Build history of the part. All positions in model axes, mm. A direction names the side the tool comes from. Give positions to 0.01 mm unless a question says otherwise; leave off trailing zeros. Write each loop counter-clockwise with the first axis right and the second up, starting at its lowest first coordinate (ties: lowest second). Pieces come first, ordered by that corner, then holes. Notation, with made-up numbers: (43, 13) -> (65, 13) arc R23 ccw to (65, 42) -> close; hole circle Ø11 at (-10, 39.25). An arc over 180 degrees is marked (long way). Put each result on its own line as item: value.
from build123d import *

# Parameters (mm, degrees)
SKETCH1_R           = 5
BOSS_EXTRUDE1_DEPTH = 10
SKETCH2_W           = 60
SKETCH2_H           = 40
BOSS_EXTRUDE2_DEPTH = 30
SKETCH3_W           = 60
SKETCH3_H           = 40
BOSS_EXTRUDE3_DEPTH = 20


with BuildPart() as part:
    # Sketch1 → Boss-Extrude1 (new body)
    with BuildSketch(Plane.XY):
        with BuildLine():
            Line((-30, -15), (-30, -20))
            Line((-30, -20), (30, -20))
            Line((30, -20), (30, 20))
            Line((30, 20), (-30, 20))
            Line((-30, 20), (-30, 15))
            Line((-30, 15), (-50, 15))
            ThreePointArc((-50, 15), (-65, 0), (-50, -15))
            Line((-50, -15), (-30, -15))
        make_face()
        with Locations((-50, 0)):
            Circle(SKETCH1_R, mode=Mode.SUBTRACT)
    extrude(amount=BOSS_EXTRUDE1_DEPTH)

    # Sketch2 → Boss-Extrude2 (add)
    with BuildSketch(Plane.XY.offset(10)):
        Rectangle(SKETCH2_W, SKETCH2_H)
    extrude(amount=BOSS_EXTRUDE2_DEPTH)

    # Sketch3 → Boss-Extrude3 (add)
    with BuildSketch(Plane(origin=(0, 0, 0), x_dir=(-1, 0, 0), z_dir=(0, 0, -1))):
        Rectangle(SKETCH3_W, SKETCH3_H)
    extrude(amount=BOSS_EXTRUDE3_DEPTH)


solid = part.part
1) Slice it at B-B (y = 13). Write the cut outline in (x, z), plus the area to 3 significant figures.
Filled sheet:
outline: (-57.48, 0) -> (-30, 0) -> (-30, -20) -> (30, -20) -> (30, 40) -> (-30, 40) -> (-30, 10) -> (-57.48, 10) -> close
area: 3,870 mm2
2) Tool access for faces 4 (the flat face through (-40, -15, 5)), 5 (the flat face through (-44, 0, 10)), 6 (the flat face through (-44, 0, 0)), 7 (the flat face through (0, -20, 10)), 8 (the flat face through (-40, 15, 5)): list every direction of +Z, -Z, +X, -X, +Y, -Y with a clear straight run to the whole face (end or side of a thin tool).
Filled sheet:
face 4: +Z, -Z, -X, -Y
face 5: +Z, -X, +Y, -Y
face 6: -Z, -X, +Y, -Y
face 7: +Z, -Z, +X, -X, -Y
face 8: +Z, -Z, -X, +Y
3) Pull direction X, two halves, no side cores. Call faces 1 (the flat face through (0, 0, 40)), 2 (the cylindrical face through (-55, 0, 5)), 3 (the flat face through (30, 0, 10)): released by +X, released by -X, zero draft, split by the parting line, or undercut.
Filled sheet:
face 1: zero draft
face 2: undercut
face 3: released by +X
4) Wall check: L1, parallel to Y at x = -50, z = 7.5; L2, parallel to X at y = -14.5, z = -11.5; L3, parallel to Z at x = -47, y = 12.5. Give the ranges that are in metal, low to high.
Filled sheet:
L1: -15 to -5, 5 to 15
L2: -30 to 30
L3: 0 to 10
5) Slice it at C-C (z = 14.5). Write the cut outline in (x, y).
Filled sheet:
outline: (-30, -20) -> (30, -20) -> (30, 20) -> (-30, 20) -> close
6) Pin check, flat tips, straight feed: pin 1 (4 mm diameter, centred on y = 4, z = 26, fed in from -X); pin 2 (8 mm diameter, centred on x = -50, y = 0, fed in from -Z) (3 decimals); pin 3 (12 mm diameter, centred on y = 5.5, z = 15, fed in from -X); pin 4 (8 mm diameter, centred on x = -43.5, z = 7, fed in from +Y). Stop position of each tip, or through.
Filled sheet:
pin 1: x = -30
pin 2: through
pin 3: x = -64.84
pin 4: y = 15
7) Slice it at D-D (x = -37). Write the cut outline in (y, z).
Filled sheet:
outline: (-15, 0) -> (15, 0) -> (15, 10) -> (-15, 10) -> close
8) Slice it at A-A (y = 0). Write the cut outline in (x, z), plus the area to 3 significant figures.
Filled sheet:
outline: (-65, 0) -> (-55, 0) -> (-55, 10) -> (-65, 10) -> close; (-45, 0) -> (-30, 0) -> (-30, -20) -> (30, -20) -> (30, 40) -> (-30, 40) -> (-30, 10) -> (-45, 10) -> close
area: 3,850 mm2
